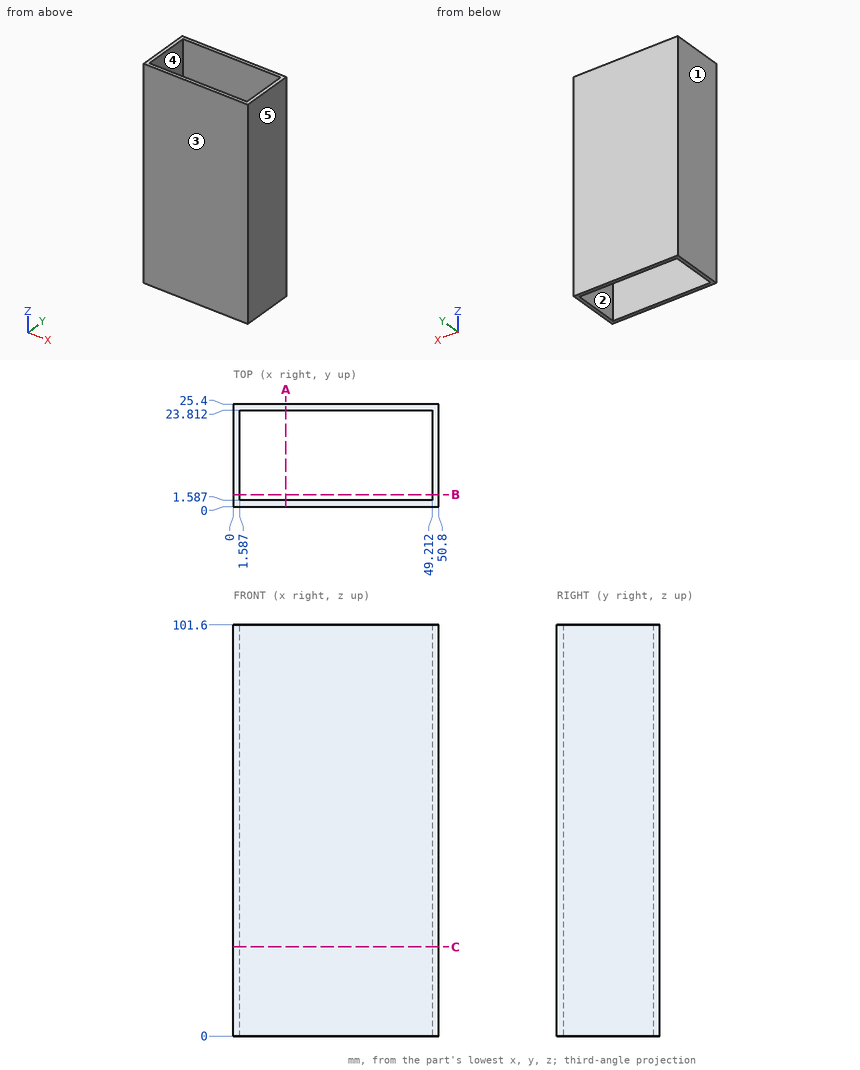
Job drawing, mm, ordinate dimensions from the low corner. One solid piece. A direction names the side the tool comes from. Coordinates: 2 decimals unless noted, no trailing zeros. Loops run counter-clockwise (first coordinate to the right, second up) from the corner with the lowest first, then second, coordinate; pieces in that order, holes last. Notation, with made-up numbers: (27.25, 0) -> (58.25, 0) arc R30 cw to (58.25, 39) -> close; hole circle Ø11 at (13.25, -29). An arc over 180 degrees is marked (long way). One line per item, written item: value.
1. Pull direction X, two halves, no side cores. Call the marked faces 3, 4 and 5: pulls with the +X half, pulls with the -X half, needs draft (parallel to the pull), parting line crosses it, or undercut.
Answers:
face 3: needs draft
face 4: undercut
face 5: pulls with the +X half
2. Drill centre lines: line 1 (X direction, y = 17.5, z = 34); line 2 (Y direction, x = 30, z = 57). Where is each one in solid material? Low to high. Write a range as [from, to].
Answers:
line 1: x = [0, 1.59], [49.21, 50.8]
line 2: y = [0, 1.59], [23.81, 25.4]
3. Slice it at C-C on z = 22. Write the cut outline in (x, y), and give its area (3 significant figures).
Answers:
outline: (0, 0) -> (50.8, 0) -> (50.8, 25.4) -> (0, 25.4) -> close; hole (1.59, 1.59) -> (49.21, 1.59) -> (49.21, 23.81) -> (1.59, 23.81) -> close
area: 232 mm^2
4. Slice it at B-B on y = 3. Write the cut outline in (x, z).
Answers:
outline: (0, 0) -> (1.59, 0) -> (1.59, 101.6) -> (0, 101.6) -> close; (49.21, 0) -> (50.8, 0) -> (50.8, 101.6) -> (49.21, 101.6) -> close
5. Flat gauge pin, fed straight in: P1, Ø5, axis at x = 45, y = 7, coming from the +Z side. Where does the tip first touch, or does it go through?
Answers:
P1: passes through
6. Slice it at A-A on x = 13. Write the cut outline in (y, z).
Answers:
outline: (0, 0) -> (1.59, 0) -> (1.59, 101.6) -> (0, 101.6) -> close; (23.81, 0) -> (25.4, 0) -> (25.4, 101.6) -> (23.81, 101.6) -> close
7. Which spindle directions (+Z, -Z, +X, -X, +Y, -Y) get a long thin tool onto all of the face, cutting with end or side? Do the marked faces 1 and 2. Say none if no direction does.
Answers:
face 1: +Z, -Z, -X, +Y, -Y
face 2: +Z, -Z
